Part model, mm, in its own coordinate system. Face numbers are marked on the shaded views. A direction names the side the tool comes from. Give positions to 0.01 mm unless a question says otherwise; leave off trailing zeros. Write each loop counter-clockwise with the first axis right and the second up, starting at its lowest first coordinate (ties: lowest second). Pieces come first, ordered by that corner, then holes. Notation, with made-up numbers: M 49,21.5 L 67,21.5 A11 cw 67,33.5 Z; hole C -19.5,72.25 d6. An arc over 180 degrees is marked long. Write item = value, one per line. Start each with the question number.
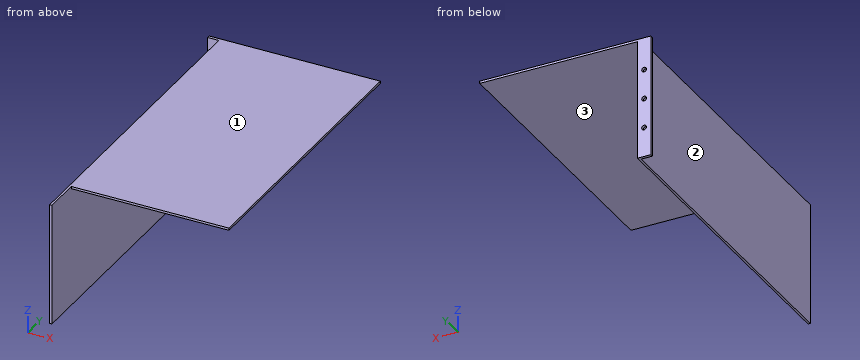
from build123d import *

# Parameters (mm, degrees)
SKETCH_1_W          = 106
SKETCH_1_H          = 195
EXTRUDE_1_DEPTH     = 1.5
SKETCH_2_W          = 82
SKETCH_2_H          = 220
EXTRUDE_2_DEPTH     = 1.5
SKETCH_3_W          = 82
SKETCH_3_H          = 2
EXTRUDE_3_DEPTH     = 9
SKETCH_5_R          = 1.6
CUT_EXTRUDE_1_DEPTH = 9


with BuildPart() as part:
    # 草图1 → 凸台-拉伸1 (new body)
    with BuildSketch(Plane.XY):
        with Locations((53, -97.5)):
            Rectangle(SKETCH_1_W, SKETCH_1_H)
    extrude(amount=EXTRUDE_1_DEPTH)

    # 草图2 → 凸台-拉伸2 (add)
    with BuildSketch(Plane.ZY):
        with Locations((-39.5, -110)):
            Rectangle(SKETCH_2_W, SKETCH_2_H)
    extrude(amount=EXTRUDE_2_DEPTH)

    # 草图3 → 凸台-拉伸3 (add)
    with BuildSketch(Plane.ZY):
        with Locations((-39.5, -1)):
            Rectangle(SKETCH_3_W, SKETCH_3_H)
    extrude(amount=EXTRUDE_3_DEPTH)

    # 草图5 → 切除-拉伸1 (cut)
    with BuildSketch(Plane(origin=(0, 0, 0), x_dir=(1, 0, 0), z_dir=(0, 1, 0))):
        with Locations(Location((-4.5, 60.5, 0), (0, 0, 270))):
            Circle(SKETCH_5_R)
        with Locations(Location((-4.5, 40.5, 0), (0, 0, 270))):
            Circle(SKETCH_5_R)
        with Locations(Location((-4.5, 20.5, 0), (0, 0, 270))):
            Circle(SKETCH_5_R)
    extrude(amount=-CUT_EXTRUDE_1_DEPTH, mode=Mode.SUBTRACT)


solid = part.part
Q1. Drop flat-ended pins along their axis: P1, Ø4, axis at y = -88, z = -71, coming from the +X side; P2, Ø3, axis at x = -4.5, z = -40.5, coming from the -Y side; P3, Ø2, axis at x = 26.5, y = -83.5, coming from the -Z side; P4, Ø1.6, axis at x = 51, z = 1, coming from the -Y side. Give the stop position or say it passes through.
Q2. Probe line 1 along X through (y, z) = (-0.8, -40.5); line 2 along Z through (x, y) = (96, -30); line 3 along X through (y, z) = (-131.5, -26). List the from-to ranges inside material, lowest first.
Q3. Slice it at B-B (z = -50). Give the cut face in (x, y).
Q4. Slice it at A-A (y = -29.5). Give the cut face in (x, z), and give its area (3 significant figures).
Q5. Tool access for the marked faces 1, 2 and 3: list every direction of +Z, -Z, +X, -X, +Y, -Y with a clear straight run to the whole face (end or side of a thin tool).
Q6. Slice it at C-C (x = 48). Give the cut face in (y, z).
Working result:
q1.P1 = 0
q1.P2 = through
q1.P3 = 0
q1.P4 = -195
q2.line_1 = -9 to -6.1, -2.9 to 0
q2.line_2 = 0 to 1.5
q2.line_3 = -1.5 to 0
q3.outline = M -9,-2 L -1.5,-2 L -1.5,-220 L 0,-220 L 0,0 L -9,0 Z
q4.outline = M -1.5,-80.5 L 0,-80.5 L 0,0 L 106,0 L 106,1.5 L -1.5,1.5 Z
q4.area = 282 mm2
q5.face_1 = +Z, +X, -X, +Y, -Y
q5.face_2 = +Z, -Z, -X, -Y
q5.face_3 = -Z, +X, +Y, -Y
q6.outline = M -195,0 L 0,0 L 0,1.5 L -195,1.5 Z
